For this review, take the finished solid that the model builds, in its own axes (mm). Face numbers are marked on the shaded views. A direction names the side the tool comes from. Coordinates: 2 decimals unless noted, no trailing zeros. Loops run counter-clockwise (first coordinate to the right, second up) from the corner with the lowest first, then second, coordinate; pieces in that order, holes last.
1. Machinability: for the marked faces 5, 6, 7 and 8, which of the approach directions +Z, -Z, +X, -X, +Y, -Y give a long, thin tool a straight path to every point of the face, cutting with its end or side? Answer none if there is none.
2. Clearance check with flat-ended pins moving along their axes: P1, Ø12, axis at x = 9, z = 7, coming from the -Y side; P2, Ø1.5, axis at x = 19.5, y = 21.5, coming from the +Z side; P3, Ø12.5, axis at y = 13.5, z = 22.5, coming from the -X side; P4, Ø8.5, axis at y = 8, z = 14, coming from the +X side. State where each tip first meets the part, or that it passes through.
3. Take a section at A-A, the plane x = 27.5. State the section outline as (y, z) points.
4. Mouldability with a two-part tool opening along X and no side actions: class the marked faces 1, 2, 3 and 4 as pulls with the +X half, pulls with the -X half, needs draft (parallel to the pull), parting line crosses it, or undercut.
5. Take a section at B-B, the plane y = 17. State the section outline as (x, z) points.
6. Take a section at C-C, the plane z = 14. State the section outline as (x, y) points, then the cut area to 3 significant figures.
7. Take a section at D-D, the plane y = 25.5. State the section outline as (x, z) points.
8. To check wall thickness, follow probe 1 along X at (y, z) = (0.5, 4); probe 2 along Z at (x, y) = (2.5, 18); probe 3 along X at (y, z) = (23, 30). State the ranges of each line that lie inside material, in increasing order.
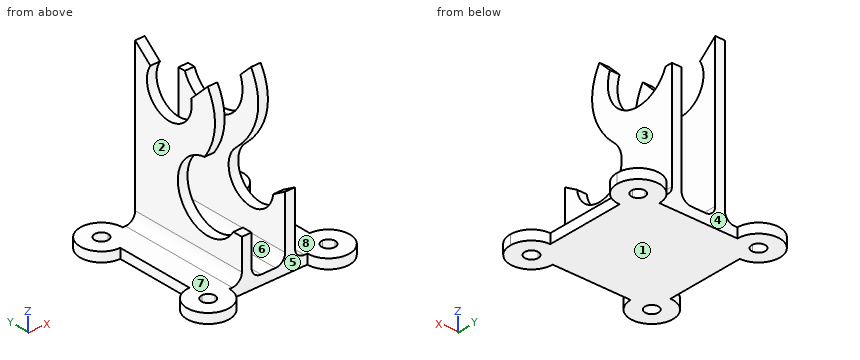
```python
from build123d import *

# Parameters (mm, degrees)
SKETCH1_W           = 3.5
SKETCH1_H           = 25
BOSS_EXTRUDE1_DEPTH = 2
SKETCH1_3_W         = 2
SKETCH1_3_H         = 25
BOSS_EXTRUDE2_DEPTH = 40
CUT_EXTRUDE12_REACH = 56.462
SKETCH2_R           = 5.25
SKETCH2_R_2         = 7
CUT_EXTRUDE13_REACH = 56.462
SKETCH3_R           = 5.25
SKETCH3_R_2         = 7
CUT_EXTRUDE14_DEPTH = 55.462096912
CUT_EXTRUDE15_REACH = 52.769
SKETCH6_W           = 4.605551275
SKETCH6_H           = 2
CUT_EXTRUDE16_REACH = 52.769
FILLET1_R           = 2


with BuildPart() as part:
    # Sketch1 → Boss-Extrude1 (new body)
    with BuildSketch(Plane.XY):
        with BuildLine():
            ThreePointArc((0, 20.6), (3.111269837, 21.888730163), (4.4, 25))
            Line((4.4, 25), (1.4, 25))
            ThreePointArc((1.4, 25), (0.989949494, 24.010050506), (0, 23.6))
            Line((0, 23.6), (0, 20.6))
        make_face()
        with BuildLine():
            Line((1.4, 25), (4.4, 25))
            ThreePointArc((4.4, 25), (-3.111269837, 28.111269837), (0, 20.6))
            Line((0, 20.6), (0, 23.6))
            ThreePointArc((0, 23.6), (-0.989949494, 25.989949494), (1.4, 25))
        make_face()
        with BuildLine():
            Line((7, 0), (7, 25))
            Line((7, 25), (4.4, 25))
            ThreePointArc((4.4, 25), (3.111269837, 21.888730163), (0, 20.6))
            Line((0, 20.6), (0, 4.4))
            ThreePointArc((0, 4.4), (3.111269837, 3.111269837), (4.4, 0))
            Line((4.4, 0), (7, 0))
        make_face()
        with BuildLine():
            ThreePointArc((0, 4.4), (-3.111269837, -3.111269837), (4.4, 0))
            Line((4.4, 0), (1.4, 0))
            ThreePointArc((1.4, 0), (-0.989949494, -0.989949494), (0, 1.4))
            Line((0, 1.4), (0, 4.4))
        make_face()
        with BuildLine():
            Line((1.4, 0), (4.4, 0))
            ThreePointArc((4.4, 0), (3.111269837, 3.111269837), (0, 4.4))
            Line((0, 4.4), (0, 1.4))
            ThreePointArc((0, 1.4), (0.989949494, 0.989949494), (1.4, 0))
        make_face()
        with Locations((10.75, 12.5)):
            Rectangle(SKETCH1_W, SKETCH1_H)
        with Locations((14.25, 12.5)):
            Rectangle(SKETCH1_W, SKETCH1_H)
        with BuildLine():
            Line((20.6, 25), (18, 25))
            Line((18, 25), (18, 0))
            Line((18, 0), (20.6, 0))
            ThreePointArc((20.6, 0), (21.888730163, 3.111269837), (25, 4.4))
            Line((25, 4.4), (25, 20.6))
            ThreePointArc((25, 20.6), (21.888730163, 21.888730163), (20.6, 25))
        make_face()
        with BuildLine():
            ThreePointArc((29.4, 25), (25, 29.4), (20.6, 25))
            Line((20.6, 25), (23.6, 25))
            ThreePointArc((23.6, 25), (25, 26.4), (26.4, 25))
            ThreePointArc((26.4, 25), (25.989949494, 24.010050506), (25, 23.6))
            Line((25, 23.6), (25, 20.6))
            ThreePointArc((25, 20.6), (28.111269837, 21.888730163), (29.4, 25))
        make_face()
        with BuildLine():
            Line((23.6, 25), (20.6, 25))
            ThreePointArc((20.6, 25), (21.888730163, 21.888730163), (25, 20.6))
            Line((25, 20.6), (25, 23.6))
            ThreePointArc((25, 23.6), (24.010050506, 24.010050506), (23.6, 25))
        make_face()
        with BuildLine():
            ThreePointArc((25, 4.4), (21.888730163, 3.111269837), (20.6, 0))
            Line((20.6, 0), (23.6, 0))
            ThreePointArc((23.6, 0), (24.010050506, 0.989949494), (25, 1.4))
            Line((25, 1.4), (25, 4.4))
        make_face()
        with BuildLine():
            Line((23.6, 0), (20.6, 0))
            ThreePointArc((20.6, 0), (25, -4.4), (29.4, 0))
            ThreePointArc((29.4, 0), (28.111269837, 3.111269837), (25, 4.4))
            Line((25, 4.4), (25, 1.4))
            ThreePointArc((25, 1.4), (25.989949494, 0.989949494), (26.4, 0))
            ThreePointArc((26.4, 0), (25, -1.4), (23.6, 0))
        make_face()
    extrude(amount=BOSS_EXTRUDE1_DEPTH)

    # Sketch1_3 → Boss-Extrude2 (add)
    with BuildSketch(Plane.XY):
        with Locations((8, 12.5)):
            Rectangle(SKETCH1_3_W, SKETCH1_3_H)
        with Locations((17, 12.5)):
            Rectangle(SKETCH1_3_W, SKETCH1_3_H)
    extrude(amount=BOSS_EXTRUDE2_DEPTH)

    # Sketch2 → Cut-Extrude12 (cut, up to next)
    with BuildSketch(Plane.ZY.offset(-7), mode=Mode.PRIVATE) as cut_extrude12_sk1:
        with Locations(Location((29, 17, 0), (0, 0, 270))):
            Circle(SKETCH2_R)
    cut_extrude12_tool1 = extrude(cut_extrude12_sk1.sketch, amount=-CUT_EXTRUDE12_REACH, mode=Mode.PRIVATE) & part.part
    # Sketch2 → Cut-Extrude12 (cut, up to next)
    with BuildSketch(Plane.ZY.offset(-7), mode=Mode.PRIVATE) as cut_extrude12_sk2:
        with Locations(Location((14, 8, 0), (0, 0, 270))):
            Circle(SKETCH2_R_2)
    cut_extrude12_tool2 = extrude(cut_extrude12_sk2.sketch, amount=-CUT_EXTRUDE12_REACH, mode=Mode.PRIVATE) & part.part
    add(cut_extrude12_tool1.solids().sort_by_distance((7, 17, 29))[0], mode=Mode.SUBTRACT)
    add(cut_extrude12_tool2.solids().sort_by_distance((7, 8, 14))[0], mode=Mode.SUBTRACT)

    # Sketch3 → Cut-Extrude13 (cut, up to next)
    with BuildSketch(Plane(origin=(18, 0, 0), x_dir=(0, 0, -1), z_dir=(1, 0, 0)), mode=Mode.PRIVATE) as cut_extrude13_sk1:
        with Locations(Location((-14, 8, 0), (0, 0, 90))):
            Circle(SKETCH3_R)
    cut_extrude13_tool1 = extrude(cut_extrude13_sk1.sketch, amount=-CUT_EXTRUDE13_REACH, mode=Mode.PRIVATE) & part.part
    # Sketch3 → Cut-Extrude13 (cut, up to next)
    with BuildSketch(Plane(origin=(18, 0, 0), x_dir=(0, 0, -1), z_dir=(1, 0, 0)), mode=Mode.PRIVATE) as cut_extrude13_sk2:
        with Locations(Location((-29, 17, 0), (0, 0, 90))):
            Circle(SKETCH3_R_2)
    cut_extrude13_tool2 = extrude(cut_extrude13_sk2.sketch, amount=-CUT_EXTRUDE13_REACH, mode=Mode.PRIVATE) & part.part
    add(cut_extrude13_tool1.solids().sort_by_distance((18, 8, 14))[0], mode=Mode.SUBTRACT)
    add(cut_extrude13_tool2.solids().sort_by_distance((18, 17, 29))[0], mode=Mode.SUBTRACT)

    # Sketch5 → Cut-Extrude14 (cut, through all)
    with BuildSketch(Plane.ZY.offset(-7)):
        with BuildLine():
            Line((31.804811412, 21.437964955), (34.804811412, 25))
            Line((34.804811412, 25), (40, 25))
            Line((40, 25), (40, 0))
            Line((40, 0), (15, 0))
            Line((15, 0), (13.312046989, 2.795269397))
            Line((13.312046989, 2.795269397), (18.15476351, 11.209429883))
            add(Edge.make_bspline(
                [(34, 8), (28.19172845, 4.568111712), (22.349790319, 6.720692965), (18.15476351, 11.209429883)],
                knots=[0, 0, 0, 0, 1, 1, 1, 1], degree=3))
            Line((34, 8), (30.135621564, 11.874293838))
            Line((30.135621564, 11.874293838), (31.804811412, 21.437964955))
        make_face()
    extrude(amount=-CUT_EXTRUDE14_DEPTH, mode=Mode.SUBTRACT)

    # Sketch6 → Cut-Extrude15 (cut, up to next)
    with BuildSketch(Plane.ZY.offset(-7), mode=Mode.PRIVATE) as cut_extrude15_sk1:
        with Locations((12.697224363, 1)):
            Rectangle(SKETCH6_W, SKETCH6_H)
    cut_extrude15_tool1 = extrude(cut_extrude15_sk1.sketch, amount=-CUT_EXTRUDE15_REACH, mode=Mode.PRIVATE) & part.part
    add(cut_extrude15_tool1.solids().sort_by_distance((7, 1, 12.697224))[0], mode=Mode.SUBTRACT)

    # Sketch7 → Cut-Extrude16 (cut, up to next)
    with BuildSketch(Plane(origin=(18, 0, 0), x_dir=(0, 0, -1), z_dir=(1, 0, 0)), mode=Mode.PRIVATE) as cut_extrude16_sk1:
        with BuildLine():
            Line((-34.804811412, 25), (-26.401923789, 25))
            Line((-26.401923789, 25), (-26.401923789, 23.5))
            ThreePointArc((-26.401923789, 23.5), (-30.6033676, 19.298556189), (-34.804811412, 23.5))
            Line((-34.804811412, 23.5), (-34.804811412, 25))
        make_face()
    cut_extrude16_tool1 = extrude(cut_extrude16_sk1.sketch, amount=-CUT_EXTRUDE16_REACH, mode=Mode.PRIVATE) & part.part
    add(cut_extrude16_tool1.solids().sort_by_distance((18, 22.508493, 30.603368))[0], mode=Mode.SUBTRACT)

    # Fillet1
    fillet1_edges = [part.edges().sort_by_distance(p)[0] for p in [
        (7, 12.5, 2),
        (16, 12.5, 2),
        (9, 12.5, 2),
        (18, 12.5, 2),
    ]]
    fillet(fillet1_edges, radius=FILLET1_R)


solid = part.part
```
Results list:
1. face 5: +Z, -Z, -Y
1. face 6: +Z, +Y, -Y
1. face 7: +Z, -X, +Y, -Y
1. face 8: +Z, +X, +Y, -Y
2. P1: stops at y = 0
2. P2: stops at z = 2.44
2. P3: stops at x = 7
2. P4: passes through
3. outline: (-3.62, 0) - (3.62, 0) - (3.62, 2) - (-3.62, 2) - close; (21.38, 0) - (28.62, 0) - (28.62, 2) - (21.38, 2) - close
4. face 1: needs draft
4. face 2: pulls with the -X half
4. face 3: pulls with the +X half
4. face 4: undercut
5. outline: (0, 0) - (25, 0) - (25, 2) - (20, 2) arc R2 cw to (18, 4) - (18, 22) - (16, 22) - (16, 4) arc R2 cw to (14, 2) - (11, 2) arc R2 cw to (9, 4) - (9, 23.75) - (7, 23.75) - (7, 4) arc R2 cw to (5, 2) - (0, 2) - close
6. outline: (7, 15) - (9, 15) - (9, 25) - (7, 25) - close; (16, 0) - (18, 0) - (18, 1.66) - (16, 1.66) - close; (16, 13.25) - (18, 13.25) - (18, 25) - (16, 25) - close
6. area: 46.8 mm2
7. outline: (-4.37, 0) - (-1.31, 0) - (-1.31, 2) - (-4.37, 2) - close; (1.31, 0) - (4.37, 0) - (4.37, 2) - (1.31, 2) - close; (20.63, 0) - (23.69, 0) - (23.69, 2) - (20.63, 2) - close; (26.31, 0) - (29.37, 0) - (29.37, 2) - (26.31, 2) - close
8. probe 1: x = 7 to 9, 16 to 18
8. probe 2: z = 0 to 2
8. probe 3: x = 7 to 9
